CAD build for the part. Positions are in the model's coordinates, mm. A direction names the side the tool comes from. Coordinates: 2 decimals unless noted, no trailing zeros. Write each loop counter-clockwise with the first axis right and the second up, starting at its lowest first coordinate (ties: lowest second). Pieces come first, ordered by that corner, then holes. Notation, with made-up numbers: (50.25, -38.5) - (95.25, -38.5) arc R35 cw to (95.25, -3.5) - close; hole circle Ø5 at (24.5, 5.25). An arc over 180 degrees is marked (long way). One line per question, with ' | ' between items. Start each with the question number.
1. Band-saw the part on B-B, the plane y = 0. Write the cut outline in (x, z).
2. Probe line 1 (Y direction, x = -0.1, z = 3.25); line 2 (Y direction, x = -1.25, z = -3.25); line 3 (Z direction, x = 0.55, y = -2.5). List the from-to ranges inside material, lowest first.
3. Band-saw the part on C-C, the plane z = -1. Write the cut outline in (x, y).
4. Two-plate mould, pull along Z, no slides. Class faces 1 (the flat face through (-2, 2, 1)), 2 (the flat face through (-2, 2, 2)), 3 (the cylindrical face through (-3, 0.1, 1.5)): +Z half, -Z half, draft (parallel to the pull), parting line (faces both ways), or undercut.
5. Which spindle directions (+Z, -Z, +X, -X, +Y, -Y) get a long thin tool onto all of the face, cutting with end or side? Do faces 4 (the cylindrical face through (2.75, -0.03, -3.94)), 5 (the cylindrical face through (-2.75, 0.03, -3.94)), 6 (the cylindrical face through (0.54, 2.44, 0.49)), 7 (the flat face through (0, -1.887, -4)). Say none if no direction does.
6. Band-saw the part on A-A, the plane x = 0. Write the cut outline in (y, z), then the cut area to 3 significant figures.
7. Band-saw the part on D-D, the plane y = 2.2. Write the cut outline in (x, z).
8. Flat gauge pins, fed straight in: P1, Ø2, axis at y = -0.5, z = 5, coming from the +X side; P2, Ø2, axis at x = 0, z = -4.5, coming from the -Y side; P3, Ø1.2, axis at x = 0, z = -5.5, coming from the +Y side. Where does each tip first touch, or does it go through?
from build123d import *

# Parameters (mm, degrees)
SKETCH_1_R      = 2.5
EXTRUDE_1_DEPTH = 6.2
EXTRUDE_2_DEPTH = 8
SKETCH_3_R      = 2.5
EXTRUDE_3_DEPTH = 0.8
EXTRUDE_START   = 1
SKETCH_4_R      = 3
EXTRUDE_4_DEPTH = 1


with BuildPart() as part:
    # 草图1 → 凸台-拉伸1 (new body)
    with BuildSketch(Plane.XY):
        with Locations(Location((0, 0, 0), (0, 0, 180))):
            Circle(SKETCH_1_R)
    extrude(amount=EXTRUDE_1_DEPTH)

    # 草图2 → 凸台-拉伸2 (add)
    with BuildSketch(Plane(origin=(0, 0, 0), x_dir=(-1, 0, 0), z_dir=(0, 0, -1))):
        with BuildLine():
            Line((-2, 1.887458609), (2, 1.887458609))
            ThreePointArc((2, 1.887458609), (2.75, 0), (2, -1.887458609))
            Line((2, -1.887458609), (-2, -1.887458609))
            ThreePointArc((-2, -1.887458609), (-2.75, 0), (-2, 1.887458609))
        make_face()
    extrude(amount=EXTRUDE_2_DEPTH)

    # 草图3 → 凸台-拉伸3 (add)
    with BuildSketch(Plane.XY.offset(6.2)):
        with Locations(Location((0, 0, 0), (0, 0, 130.976076876))):
            Circle(SKETCH_3_R)
    extrude(amount=EXTRUDE_3_DEPTH)

    # 草图4 → 凸台-拉伸4 (add)
    with BuildSketch(Plane.XY.offset(EXTRUDE_START)):
        Circle(SKETCH_4_R)
    extrude(amount=EXTRUDE_4_DEPTH)


solid = part.part
Filled in:
1) outline: (-3, 1) - (-2.5, 1) - (-2.5, 0) - (-2.75, 0) - (-2.75, -8) - (2.75, -8) - (2.75, 0) - (2.5, 0) - (2.5, 1) - (3, 1) - (3, 2) - (2.5, 2) - (2.5, 7) - (-2.5, 7) - (-2.5, 2) - (-3, 2) - close
2) line 1: y = -2.5 to 2.5 | line 2: y = -1.89 to 1.89 | line 3: z = 1 to 2
3) outline: (-2, -1.89) - (2, -1.89) arc R2.75 ccw to (2, 1.89) - (-2, 1.89) arc R2.75 ccw to start
4) face 1: undercut | face 2: +Z half | face 3: draft
5) face 4: -Z, +X | face 5: -Z, -X | face 6: none | face 7: -Z, +X, -X, -Y
6) outline: (-3, 1) - (-2.5, 1) - (-2.5, 0) - (-1.89, 0) - (-1.89, -8) - (1.89, -8) - (1.89, 0) - (2.5, 0) - (2.5, 1) - (3, 1) - (3, 2) - (2.5, 2) - (2.5, 7) - (-2.5, 7) - (-2.5, 2) - (-3, 2) - close | area: 66.2 mm²
7) outline: (-2.04, 1) - (-1.19, 1) - (-1.19, 0) - (1.19, 0) - (1.19, 1) - (2.04, 1) - (2.04, 2) - (1.19, 2) - (1.19, 7) - (-1.19, 7) - (-1.19, 2) - (-2.04, 2) - close
8) P1: stops at x = 2.5 | P2: stops at y = -1.89 | P3: stops at y = 1.89
